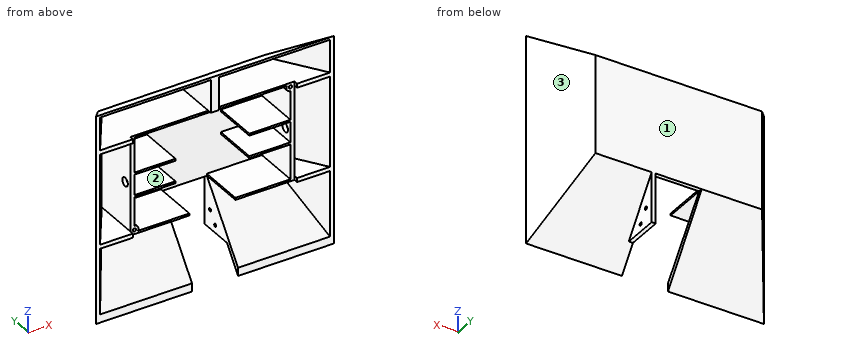
from build123d import *

# Parameters (mm, degrees)
CUT_EXTRUDE3_START      = -32.5
SKETCH7_W               = 100
SKETCH7_H               = 60
CUT_EXTRUDE3_DEPTH      = 30
CUT_EXTRUDE6_DEPTH      = 14
CUT_EXTRUDE6_DEPTH_BACK = 14
BOSS_EXTRUDE1_DEPTH     = 2.5
BOSS_EXTRUDE2_DEPTH     = 30
BOSS_EXTRUDE3_START     = -2.5
BOSS_EXTRUDE3_DEPTH     = 5
BOSS_EXTRUDE4_START     = -30
BOSS_EXTRUDE4_DEPTH     = 2.5
BOSS_EXTRUDE4_START_2   = 27.5
BOSS_EXTRUDE4_2_DEPTH   = 2.5
BOSS_EXTRUDE5_START     = -30
BOSS_EXTRUDE5_DEPTH     = 2.5
BOSS_EXTRUDE5_START_2   = 27.5
BOSS_EXTRUDE5_2_DEPTH   = 2.5
SKETCH20_W              = 100
SKETCH20_H              = 60
CUT_EXTRUDE7_DEPTH      = 2.5
CUT_EXTRUDE8_START      = -2.5
SKETCH21_R              = 2.627
CUT_EXTRUDE8_DEPTH      = 100
SKETCH13_R              = 1
CUT_EXTRUDE9_DEPTH      = 2.5
CUT_EXTRUDE11_START     = -1.2
SKETCH23_W              = 181.319522923
SKETCH23_H              = 53.809633396
CUT_EXTRUDE11_DEPTH     = 4
SKETCH24_R              = 2.5
BOSS_EXTRUDE6_DEPTH     = 2.5
SKETCH25_R              = 1
CUT_EXTRUDE12_DEPTH     = 2.5
CUT_EXTRUDE13_START     = -2
SKETCH26_W              = 145.47086515
SKETCH26_H              = 58.938684545
CUT_EXTRUDE13_DEPTH     = 2.5
CUT_EXTRUDE14_START     = -2
SKETCH27_W              = 157.368673289
SKETCH27_H              = 83.270010287
CUT_EXTRUDE14_DEPTH     = 2.5


# Read off the part's stored shape, not the designer's step: Boss-Extrude3, Boss-Extrude4, Boss-Extrude5
with BuildPart() as part:
    # Sketch1 → Loft1 section 0
    with BuildSketch(Plane(origin=(0, 0, 0), x_dir=(1, 0, 0), z_dir=(0, 1, 0))):
        with BuildLine():
            Line((-75, -55), (-75, 75))
            Line((-75, 75), (75, 75))
            Line((75, 75), (75, -55))
            Line((75, -55), (-75, -55))
        make_face()
    # Sketch2 → Loft1 section 1
    with BuildSketch(Plane(origin=(0, 32.5, 0), x_dir=(1, 0, 0), z_dir=(0, 1, 0))):
        with BuildLine():
            Line((-52.5, -30), (52.5, -30))
            Line((52.5, -30), (52.5, 30))
            Line((52.5, 30), (-52.5, 30))
            Line((-52.5, 30), (-52.5, -30))
        make_face()
    loft()

    # Sketch7 → Cut-Extrude3 (cut)
    with BuildSketch(Plane(origin=(0, 32.5, 0), x_dir=(1, 0, 0), z_dir=(0, 1, 0)).offset(CUT_EXTRUDE3_START)):
        Rectangle(SKETCH7_W, SKETCH7_H)
    extrude(amount=CUT_EXTRUDE3_DEPTH, mode=Mode.SUBTRACT)

    # Sketch8 → Cut-Extrude6 (cut, two sides: drawn at the far end of the back side and taken through both)
    with BuildSketch(Plane(origin=(0, 0, 0), x_dir=(0, 0, -1), z_dir=(1, 0, 0)).offset(-CUT_EXTRUDE6_DEPTH_BACK)):
        Polygon((30, 35.583833793), (79.269923714, 0), (30, 0), align=None)
    extrude(amount=CUT_EXTRUDE6_DEPTH + CUT_EXTRUDE6_DEPTH_BACK, mode=Mode.SUBTRACT)

    # Sketch11 → Cut-Loft1 section 0
    with BuildSketch(Plane.XZ.offset(-30)):
        with BuildLine():
            Line((-50, 30), (50, 30))
            Line((50, 30), (50, -30))
            Line((50, -30), (-50, -30))
            Line((-50, -30), (-50, 30))
        make_face()
    # Sketch9 → Cut-Loft1 section 1
    with BuildSketch(Plane.XZ):
        with BuildLine():
            Line((-70, 50), (70, 50))
            Line((70, 50), (70, -70))
            Line((70, -70), (-70, -70))
            Line((-70, -70), (-70, 50))
        make_face()
    loft(mode=Mode.SUBTRACT)

    # Sketch12 → Boss-Extrude1 (add)
    with BuildSketch(Plane.ZY.offset(-14)):
        Polygon((-60.5, 32.5), (-60.5, 10.472222222), (-30, 32.5), align=None)
    extrude(amount=-BOSS_EXTRUDE1_DEPTH)

    # Sketch14 → Boss-Extrude2 (add)
    with BuildSketch(Plane.XZ.offset(-30)):
        Polygon((-50, -30), (-50, 30), (50, 30), (50, -30), (14, -30), (14, -28.75), (47.5, -28.75), (47.5, -7.5), (22.5, -7.5), (22.5, -6.25), (47.5, -6.25), (47.5, 6.25), (22.5, 6.25), (22.5, 7.5), (47.5, 7.5), (47.5, 28.75), (-47.5, 28.75), (-47.5, 7.5), (-22.5, 7.5), (-22.5, 6.25), (-47.5, 6.25), (-47.5, -6.25), (-22.5, -6.25), (-22.5, -7.5), (-47.5, -7.5), (-47.5, -28.75), (-14, -28.75), (-14, -30), (-47.5, -30), align=None)
    extrude(amount=BOSS_EXTRUDE2_DEPTH)

    # Boss-Extrude3 outline → Boss-Extrude3 (add)
    with BuildSketch(Plane.YZ.offset(BOSS_EXTRUDE3_START)):
        Polygon((30, 30), (0, 50), (0, 30), align=None)
    extrude(amount=BOSS_EXTRUDE3_DEPTH)

    # Boss-Extrude4 outline → Boss-Extrude4 (add)
    with BuildSketch(Plane.XY.offset(BOSS_EXTRUDE4_START)):
        Polygon((-50, 30), (-70, 0), (-50, 0), align=None)
    extrude(amount=BOSS_EXTRUDE4_DEPTH)

    # Boss-Extrude4 2 outline → Boss-Extrude4 2 (add)
    with BuildSketch(Plane.XY.offset(BOSS_EXTRUDE4_START_2)):
        Polygon((-50, 30), (-70, 0), (-50, 0), align=None)
    extrude(amount=BOSS_EXTRUDE4_2_DEPTH)

    # Boss-Extrude5 outline → Boss-Extrude5 (add)
    with BuildSketch(Plane.XY.offset(BOSS_EXTRUDE5_START)):
        Polygon((50, 30), (50, 0), (70, 0), align=None)
    extrude(amount=BOSS_EXTRUDE5_DEPTH)

    # Boss-Extrude5 2 outline → Boss-Extrude5 2 (add)
    with BuildSketch(Plane.XY.offset(BOSS_EXTRUDE5_START_2)):
        Polygon((50, 30), (50, 0), (70, 0), align=None)
    extrude(amount=BOSS_EXTRUDE5_2_DEPTH)

    # Sketch20 → Cut-Extrude7 (cut)
    with BuildSketch(Plane.XZ):
        Rectangle(SKETCH20_W, SKETCH20_H)
    extrude(amount=-CUT_EXTRUDE7_DEPTH, mode=Mode.SUBTRACT)

    # Sketch21 → Cut-Extrude8 (cut)
    with BuildSketch(Plane(origin=(-47.5, 0, 0), x_dir=(0, 0, -1), z_dir=(1, 0, 0)).offset(CUT_EXTRUDE8_START)):
        with Locations(Location((0, 7.5, 0), (0, 0, 180))):
            Circle(SKETCH21_R)
    extrude(amount=CUT_EXTRUDE8_DEPTH, mode=Mode.SUBTRACT)

    # Sketch13 → Cut-Extrude9 (cut)
    with BuildSketch(Plane(origin=(16.5, 0, 0), x_dir=(0, 0, -1), z_dir=(1, 0, 0))):
        with Locations((55.923446724, 21.955394633)):
            Circle(SKETCH13_R)
        with Locations((49.044605367, 26.923446724)):
            Circle(SKETCH13_R)
    extrude(amount=-CUT_EXTRUDE9_DEPTH, mode=Mode.SUBTRACT)

    # Sketch23 → Cut-Extrude11 (cut)
    with BuildSketch(Plane(origin=(0, 23.076923077, 34.615384615), x_dir=(-1, 0, 0), z_dir=(0, -0.5547001962252286, -0.8320502943378442)).offset(CUT_EXTRUDE11_START)):
        with Locations((-1.646246513, -10.343211106)):
            Rectangle(SKETCH23_W, SKETCH23_H)
    extrude(amount=-CUT_EXTRUDE11_DEPTH, mode=Mode.SUBTRACT)

    # Sketch24 → Boss-Extrude6 (add)
    with BuildSketch(Plane.XZ.offset(-2.5)):
        with Locations((-47.5, -27.5)):
            Circle(SKETCH24_R)
        with Locations((47.5, 27.5)):
            Circle(SKETCH24_R)
    extrude(amount=-BOSS_EXTRUDE6_DEPTH)

    # Sketch25 → Cut-Extrude12 (cut)
    with BuildSketch(Plane.XZ.offset(-2.5)):
        with Locations(Location((-47.5, -27.5, 0), (0, 0, 270))):
            Circle(SKETCH25_R)
        with Locations(Location((47.5, 27.5, 0), (0, 0, 270))):
            Circle(SKETCH25_R)
    extrude(amount=-CUT_EXTRUDE12_DEPTH, mode=Mode.SUBTRACT)

    # Sketch26 → Cut-Extrude13 (cut)
    with BuildSketch(Plane(origin=(-48.461538462, 32.307692308, 0), x_dir=(0, 0, -1), z_dir=(0.8320502943378436, -0.5547001962252295, 0)).offset(CUT_EXTRUDE13_START)):
        with Locations((11.121253107, -16.230406727)):
            Rectangle(SKETCH26_W, SKETCH26_H)
    extrude(amount=-CUT_EXTRUDE13_DEPTH, mode=Mode.SUBTRACT)

    # Sketch27 → Cut-Extrude14 (cut)
    with BuildSketch(Plane(origin=(48.461538462, 32.307692308, 0), x_dir=(0, 0, 1), z_dir=(-0.8320502943378442, -0.5547001962252287, 0)).offset(CUT_EXTRUDE14_START)):
        with Locations((-8.576197042, -8.380711465)):
            Rectangle(SKETCH27_W, SKETCH27_H)
    extrude(amount=-CUT_EXTRUDE14_DEPTH, mode=Mode.SUBTRACT)


solid = part.part
Verification items for the finished model (mm, model axes). Face numbers are marked on the shaded views. Give positions to 0.01 mm unless a question says otherwise; leave off trailing zeros. Answer as a JSON object with one key per item and string values. Group by question number.
1) Cross-section at A-A (z = 0). Give the number of separate pieces and of enclosed holes in the cut face, then the cut area to 3 significant figures.
2) Scan lines: line 1 along X through (y, z) = (27.5, -11.5); line 2 along X through (y, z) = (22.5, 16.5); line 3 along Z through (x, y) = (27.5, 17). Record each from-to range of solid material in increasing order. Write a range as [from, to].
3) Depth check by flat-ended pin: pin 1 Ø10 at (y, z) = (10.5, 1.5) entering from +X; pin 2 Ø10 at (y, z) = (27.5, -43) entering from +X; pin 3 Ø10 at (x, y) = (-27.5, 7.5) entering from +Z; pin 4 Ø1.6 at (y, z) = (26.92, -49.04) entering from -X. Enter the tip coordinate at first touch or a pass-through.
4) Mould release check, pull along X, two halves, no side actions. Record for the marked faces 1, 2 and 3: released by +X, released by -X, zero draft, split by the parting line, or undercut.
Result sheet:
{
 "1": {"separate pieces": "3", "enclosed holes": "0", "area": "513 mm2"},
 "2": {"line 1": "x = [-54.07, -51.67], [-50, -47.5], [47.5, 50], [51.67, 54.07]", "line 2": "x = [-57.4, -55], [-50, -47.5], [47.5, 50], [55, 57.4]", "line 3": "z = [-51.46, -47.33], [-30, -28.75], [-7.5, -6.25], [6.25, 7.5], [28.75, 30], [38.67, 40.11]"},
 "3": {"pin 1": "stops at x = 68.74", "pin 2": "stops at x = 57.4", "pin 3": "stops at z = 49.78", "pin 4": "passes through"},
 "4": {"face 1": "zero draft", "face 2": "undercut", "face 3": "released by +X"}
}
